Could you check a few things on this drawing? It's one solid part, dimensions in mm from its lowest x, y, z. A direction names the side the tool comes from. Coordinates: 2 decimals unless noted, no trailing zeros. Loops run counter-clockwise (first coordinate to the right, second up) from the corner with the lowest first, then second, coordinate; pieces in that order, holes last. Notation, with made-up numbers: M 11,23 L 35,23 A27 cw 35,42 Z; hole C 39.5,1 d8. An arc over 180 degrees is marked long. Use one line per item in the form item = value. Start each with the question number.
(1) On a 3-axis mill with a long thin cutter (end or side, diameter ignored), from which of +Z, -Z, +X, -X, +Y, -Y can I reach the whole of each face in a straight line? I mean the marked faces 1 and 2. Say none if no direction works.
(2) Imagine slicing it at A-A, the plane z = 2. Please give me the cut outline in (x, y), and give its area (3 significant figures).
(3) Will these pins go through, and if not, where does the flat tip stop? P1, Ø1.4, axis at x = 2, z = 2, coming from the -Y side; P2, Ø1, axis at y = 6.5, z = 1, coming from the -X side.
(4) Please list where these lines run through material, in increasing order: L1, parallel to X at y = 1.25, z = 2.05; L2, parallel to X at y = 3, z = 1.7.
(5) Imagine slicing it at D-D, the plane x = 0.7. Please give me the cut outline in (y, z), and give its area (3 significant figures).
(6) Thinking about a two-plate mould opening in Z: for the marked faces 3, 4, 5 and 6, which applies, +Z half, -Z half, draft (parallel to the pull), parting line (faces both ways), or undercut?
(7) Imagine slicing it at B-B, the plane x = 2. Please give me the cut outline in (y, z), and give its area (3 significant figures).
(8) Imagine slicing it at C-C, the plane y = 9. Please give me the cut outline in (x, z), and give its area (3 significant figures).
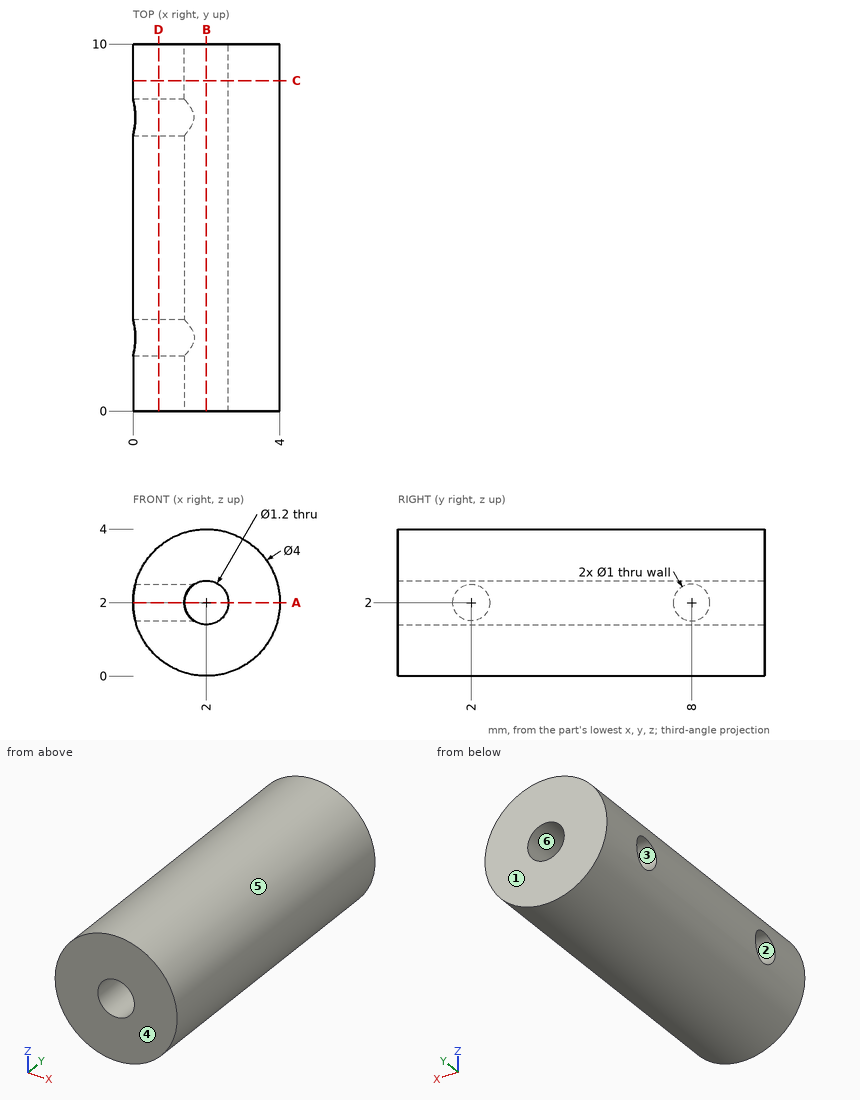
Answer:
q1.face_1 = +Z, -Z, +X, -X, +Y
q1.face_2 = -X
q2.outline = M 0,0 L 1.4,0 L 1.4,1.5 L 0,1.5 Z; M 0,2.5 L 1.4,2.5 L 1.4,7.5 L 0,7.5 Z; M 0,8.5 L 1.4,8.5 L 1.4,10 L 0,10 Z; M 2.6,0 L 4,0 L 4,10 L 2.6,10 Z
q2.area = 25.2 mm²
q3.P1 = 0
q3.P2 = 0.06
q4.L1 = 0 to 1.4, 2.6 to 4
q4.L2 = 0.02 to 1.48, 2.52 to 3.98
q5.outline = M 0,0.48 L 10,0.48 L 10,3.52 L 0,3.52 Z; hole C 2,2 d1; hole C 8,2 d1
q5.area = 28.8 mm²
q6.face_3 = undercut
q6.face_4 = draft
q6.face_5 = parting line
q6.face_6 = undercut
q7.outline = M 0,0 L 10,0 L 10,1.4 L 0,1.4 Z; M 0,2.6 L 10,2.6 L 10,4 L 0,4 Z
q7.area = 28.0 mm²
q8.outline = C 2,2 d4; hole C 2,2 d1.2
q8.area = 11.4 mm²
